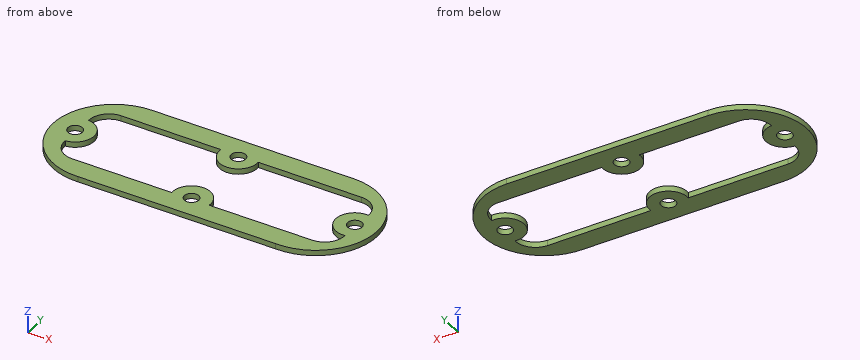
Autodesk Inventor part; units mm, degrees
ref_plane "YZ Plane" through (0, 0, 0) normal (1, 0, 0) x (0, 1, 0)
ref_plane "XZ Plane" through (0, 0, 0) normal (0, 1, 0) x (-1, 0, 0)
ref_plane "XY Plane" through (0, 0, 0) normal (0, 0, 1) x (1, 0, 0)
sketch "Sketch1" plane through (0, 0, 0) normal (0, 0, 1) x (1, 0, 0)
  line L0 (-28.1189, 16.8852) -> (28.1311, 16.8648)
  line L1 (44.9939, -0.0102) -> (44.9939, -0.0102)
  line L2 (27.4299, -16.8586) -> (-27.6697, -16.8586)
  line L3 (-45, 0.0102) -> (-45, 0.0102)
  arc A0 (-28.1189, 16.8852) -> (-27.6697, -16.8586) centre (-28.125, 0.0102) ccw
  arc A1 (27.4299, -16.8586) -> (28.1311, 16.8648) centre (28.125, -0.0041) ccw
  point P0 (0, 0)
  point P1 (-45, 16.8914)
  point P2 (45, 16.8586)
  point P3 (-45, -16.8586)
  dimension "d7" = 4
  dimension "d8" = 4
  dimension "d9" = 4
  dimension "d10" = 4
  dimension "d11" = 78
  dimension "d12" = 21
  dimension "d13" = 39
  dimension "d0" = 90
  dimension "d1" = 33.75
  dimension "d2" = 16.875
  dimension "d3" = 16.875
  dimension "d4" = 90
  dimension "d5" = 56.25
  dimension "d6" = 28.125
sketch "Sketch2" plane through (0, 0, 0) normal (0, 0, 1) x (1, 0, 0)
  circle A0 centre (-39, 0) radius 2
  circle A1 centre (39, 0) radius 2
  circle A2 centre (0, -10.5) radius 2
  circle A3 centre (0, 10.5) radius 2
  point P0 (0, 0)
  point P1 (0, 0)
  point P2 (-3.3578, 23.5)
  dimension "d7" = 4
  dimension "d8" = 4
  dimension "d9" = 4
  dimension "d10" = 4
  dimension "d11" = 78
  dimension "d12" = 21
  dimension "d13" = 39
sketch "Sketch3" plane through (0, 0, 0) normal (0, 0, 1) x (1, 0, 0)
  arc A0 (-5.2261, 11) -> (5.2261, 11) centre (0, 10.5) ccw
  arc A1 (-38.5, -5.2262) -> (-38.5, 5.2261) centre (-39, 0) ccw
  arc A2 (5.2261, -11) -> (-5.2261, -11) centre (0, -10.5) ccw
  arc A3 (39.5, 5.2261) -> (39.5, -5.2262) centre (39, 0) ccw
  line L0 (-38.5, -5.2262) -> (-38.5, -5.5)
  line L1 (-33, -11) -> (-5.2261, -11)
  line L2 (39.5, 5.2261) -> (39.5, 5.5)
  line L3 (34, 11) -> (5.2261, 11)
  line L4 (-5.2261, 11) -> (-33, 11)
  line L5 (-38.5, 5.5) -> (-38.5, 5.2261)
  line L6 (5.2261, -11) -> (34, -11)
  line L7 (39.5, -5.5) -> (39.5, -5.2262)
  arc A4 (-33, 11) -> (-38.5, 5.5) centre (-33, 5.5) ccw
  arc A5 (-38.5, -5.5) -> (-33, -11) centre (-33, -5.5) ccw
  arc A6 (39.5, 5.5) -> (34, 11) centre (34, 5.5) ccw
  arc A7 (34, -11) -> (39.5, -5.5) centre (34, -5.5) ccw
  point P0 (43.6422, -42)
  dimension "d14" = 5.5
  dimension "d15" = 5.25
  dimension "d16" = 5.25
  dimension "d17" = 5.25
  dimension "d18" = 5.25
  dimension "d19" = 22
  dimension "d20" = 78
  dimension "d23" = 5.5
  dimension "d24" = 5.5
  dimension "d25" = 5.5
  dimension "d26" = 78
extrude "Extrusion1" add sketch "Sketch1" along normal blind 1.5
extrude "Extrusion2" cut sketch "Sketch3" along normal blind 1.5
hole "Hole1" at (-39, 0, 0) at (0, 10.5, 0) at (0, -10.5, 0) at (39, 0, 0) direction (0, 0, 1) diameter 4 end through all
equation "\"d8\" = d7"
equation "\"d9\" = d7"
equation "\"d10\" = d7"
equation "\"d3\" = 0.5 * d1"
equation "\"d5\" = d0 - 2 * d3"
equation "\"d14\" = 0.5 * d21"
equation "\"d15\" = d16"
equation "\"d17\" = d16"
equation "\"d18\" = d16"
equation "\"d19\" = 2 * d21"
equation "\"d26\" = d20"
properties part number "ConnectorSeal" material "Rubber, Silicone"
Could you check a few things on this model? Use its own coordinates, in mm. Round coordinates to 2 decimals unless told otherwise and drop trailing zeros. Order: outer loops, then holes, each group sorted by start corner. A loop starts at its lowest first (then second) coordinate and runs counter-clockwise, first axis right, second up.
(1) Imagine slicing it at B-B (x = 36). Write out the boundary of the cut face in (y, z), plus the area to 3 significant figures.
Response values:
outline: (-14.92, 0) - (-10.62, 0) - (-10.62, 1.5) - (-14.92, 1.5) - close; (-4.31, 0) - (4.31, 0) - (4.31, 1.5) - (-4.31, 1.5) - close; (10.62, 0) - (14.91, 0) - (14.91, 1.5) - (10.62, 1.5) - close
area: 25.8 mm2
(2) Imagine slicing it at C-C (x = -21). Write out the boundary of the cut face in (y, z), plus the area to 3 significant figures.
Response values:
outline: (-16.86, 0) - (-11, 0) - (-11, 1.5) - (-16.86, 1.5) - close; (11, 0) - (16.88, 0) - (16.88, 1.5) - (11, 1.5) - close
area: 17.6 mm2
(3) Imagine slicing it at A-A (y = 0). Write out the boundary of the cut face in (x, z), plus the area to 3 significant figures.
Response values:
outline: (-45, 0) - (-41, 0) - (-41, 1.5) - (-45, 1.5) - close; (-37, 0) - (-33.75, 0) - (-33.75, 1.5) - (-37, 1.5) - close; (33.75, 0) - (37, 0) - (37, 1.5) - (33.75, 1.5) - close; (41, 0) - (44.99, 0) - (44.99, 1.5) - (41, 1.5) - close
area: 21.7 mm2
(4) Imagine slicing it at D-D (x = 0). Write out the boundary of the cut face in (y, z) (3 decimals), plus the area to 3 significant figures.
Response values:
outline: (-16.859, 0) - (-12.5, 0) - (-12.5, 1.5) - (-16.859, 1.5) - close; (-8.5, 0) - (-5.25, 0) - (-5.25, 1.5) - (-8.5, 1.5) - close; (5.25, 0) - (8.5, 0) - (8.5, 1.5) - (5.25, 1.5) - close; (12.5, 0) - (16.875, 0) - (16.875, 1.5) - (12.5, 1.5) - close
area: 22.9 mm2
(5) Please list where these lines run through material, in increasing order: line 1 along X through (y, z) = (0, 0.9); line 2 along Y through (x, z) = (28, 0.7); line 3 along Y through (x, z) = (-1, 1.4).
Response values:
line 1: x = -45 to -41, -37 to -33.75, 33.75 to 37, 41 to 44.99
line 2: y = -16.87 to -11, 11 to 16.86
line 3: y = -16.86 to -12.23, -8.77 to -5.35, 5.35 to 8.77, 12.23 to 16.88
(6) I'm going to push flat-ended pins straight in: pin 1 (10 mm diameter, centred on x = 17.5, y = -4.5, fed in from +Z); pin 2 (0.8 mm diameter, centred on x = 22.5, z = 1, fed in from -Y); pin 3 (4.5 mm diameter, centred on x = -39, y = 0, fed in from -Z). Where does each tip first touch, or does it pass through?
Response values:
pin 1: passes through
pin 2: stops at y = -16.86
pin 3: stops at z = 0
